Read the model definition and answer for the solid it produces. Units are mm, in the model's axes. Face numbers are marked on the shaded views. A direction names the side the tool comes from. Coordinates: 2 decimals unless noted, no trailing zeros. Loops run counter-clockwise (first coordinate to the right, second up) from the corner with the lowest first, then second, coordinate; pieces in that order, holes last. Notation, with made-up numbers: (-14.75, 86.5) -> (30.25, 86.5) arc R24 cw to (30.25, 111.5) -> close; hole circle Ø2 at (21, -30). An arc over 180 degrees is marked (long way). Answer as a JSON object with one key per item and string values. Group by question number.
Q1. The part is cut by section C-C on z = -4.25. Write down the section's boundary in (x, y) (3 decimals).
Q2. Straight lines are drawn through the part: line 1 along X through (y, z) = (-1.2, -1.5) (3 decimals); line 2 along X through (y, z) = (-0.2, -7.5) (3 decimals); line 3 along X through (y, z) = (-1.4, -7.75) (3 decimals). For each, find the intervals that lie inside material, in ascending order. Write a range as [from, to].
Q3. The part is cut by section B-B on z = -7. Write down the section's boundary in (x, y) (3 decimals), and give its area (3 significant figures).
Q4. For the marked faces 5 and 6, determine the directions among +Z, -Z, +X, -X, +Y, -Y from which every point of the face is accessible in a straight line to the end or side of a thin tool.
Q5. Determine the mould class of the marked faces 1, 2, 3 and 4 for opening direction X: released by +X, released by -X, zero draft, split by the parting line, or undercut.
Q6. The part is cut by section D-D on x = 9. Write down the section's boundary in (y, z) (3 decimals).
Q7. The part is cut by section A-A on y = -2.1. Write down the section's boundary in (x, z) (1 decimal).
Q8. Each of these flat-tipped pins is pushed along its axis until it touches: P1, Ø1.6, axis at y = -1.5, z = -6, coming from the -X side; P2, Ø8, axis at x = 6.5, z = -14, coming from the +Y side; P3, Ø3, axis at x = -3, z = -9, coming from the +Y side. Where does it stop, or does it pass through?
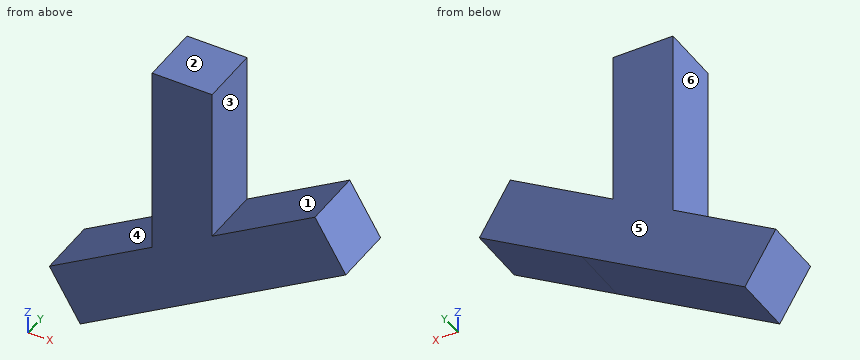
from build123d import *

# Parameters (mm, degrees)
F0_W            = 3.175
F0_H            = 10.16
F1_DEPTH        = 3.175
F2_SIZE2        = 3.17499
F2_SIZE         = 1.90499
F3_DEPTH        = 3.175
F4_DEPTH        = 6.35
F4_COPIES_COUNT = 2
F4_COPIES_PITCH = 10.052646


# Not quite as in the source:
# - a fillet or chamfer is up to 0.001 mm smaller than in the source, because OpenCascade refuses the exact size
# - a feature of the source that left no trace in its solid (it failed there, or was rolled back) is left out
# - a pattern or mirror of a feature is missing from the dataset's text; its kind, count and spacing are read off the source's solid


with BuildPart() as f1:
    # F0 (on Front) → F1 (new body)
    with BuildSketch(Plane.XZ):
        with Locations((1.5875, -5.08)):
            Rectangle(F0_W, F0_H)
    extrude(amount=F1_DEPTH)

    # F2 (size 1.905 and 3.175 in the source; OpenCascade refuses exactly that, so slightly less here)
    f2_edges = [f1.edges().sort_by_distance(p)[0] for p in [
        (3.175, -1.5875, -10.16),
    ]]
    f2_side = f1.faces().sort_by_distance((3.175, -1.5875, -5.08))[0]
    chamfer(f2_edges, length=F2_SIZE, length2=F2_SIZE2, reference=f2_side)


with BuildPart() as f3:
    # F3 (new): a face of the model
    f3_faces = [f1.part.faces().sort_by_distance(p)[0] for p in [
        (1.587505, -1.5875, -9.207505),
    ]]
    extrude(f3_faces, amount=F3_DEPTH)


with BuildPart() as f1_1:
    add(f1.part)

    # F4 (add): a face of the model
    f4_faces = [f3.part.faces().sort_by_distance(p)[0] for p in [
        (0.8167707507, -1.5875, -11.5212707762),
    ]]

    add(f3.part)  # F4 merges F3
    f4 = extrude(f4_faces, amount=F4_DEPTH)

    # F4_copies: F4 ×2
    with Locations(*[Vector(0.8574928129, 0, 0.5144959434) * (i * F4_COPIES_PITCH) for i in range(1, F4_COPIES_COUNT)]):
        add(f4)


solid = f1_1.part
Final values:
{
 "1": {"outline": "(0, -3.175) -> (3.175, -3.175) -> (3.175, 0) -> (0, 0) -> close"},
 "2": {"line 1": "x = [0, 3.175]", "line 2": "x = [0, 3.175], [4.433, 10.127]", "line 3": "x = [0, 3.175], [4.017, 10.188]"},
 "3": {"outline": "(0, -3.175) -> (3.175, -3.175) -> (3.175, 0) -> (0, 0) -> close; (5.267, -3.175) -> (9.827, -3.175) -> (9.827, 0) -> (5.267, 0) -> close", "area": "24.6 mm2"},
 "4": {"face 5": "+Z, -Z, +X, -X, +Y", "face 6": "+Z, -X, +Y, -Y"},
 "5": {"face 1": "undercut", "face 2": "zero draft", "face 3": "undercut", "face 4": "released by -X"},
 "6": {"outline": "(-3.175, -8.463) -> (0, -8.463) -> (0, -5.621) -> (-3.175, -5.621) -> close"},
 "7": {"outline": "(-5.4, -13.4) -> (-3.8, -16.1) -> (10.3, -7.7) -> (8.6, -5) -> (3.2, -8.3) -> (3.2, 0) -> (0, 0) -> (0, -10.2) -> close"},
 "8": {"P1": "stops at x = 0", "P2": "stops at y = 0", "P3": "passes through"}
}
